The model under review builds one solid part; all positions refer to its coordinate system, in mm. A direction names the side the tool comes from. Give positions to 0.01 mm unless a question says otherwise; leave off trailing zeros. Write each loop counter-clockwise with the first axis right and the second up, starting at its lowest first coordinate (ties: lowest second). Pieces come first, ordered by that corner, then holes. Notation, with made-up numbers: (54, 39) - (65, 39) arc R24 cw to (65, 66) - close; hole circle Ø5 at (-40, 1.5). An arc over 180 degrees is marked (long way). Write item = value, one per line.
```python
from build123d import *

# Parameters (mm, degrees)
F0_W      = 124
F0_H      = 240
F1_DEPTH  = 18.5
F2_R      = 39
F2_R_2    = 17.85
F3_DEPTH  = 18.501
F5_DEPTH  = 13.5
F7_R      = 3.55
F8_DEPTH  = 2.6
F9_W      = 39.5
F9_H      = 42.75
F10_DEPTH = 6.5
F11_R     = 3


with BuildPart() as f1:
    # F0 (on Front) → F1 (new body)
    with BuildSketch(Plane.XZ):
        with Locations((62, -120)):
            Rectangle(F0_W, F0_H)
    extrude(amount=F1_DEPTH)

    # F2 (on face) → F3 (cut, through all)
    with BuildSketch(Plane(origin=(0, 0, 0), x_dir=(-1, 0, 0), z_dir=(0, 1, 0))):
        with Locations((-62, -62)):
            Circle(F2_R)
        with Locations((-62, -125.85)):
            Circle(F2_R_2)
    extrude(amount=-F3_DEPTH, mode=Mode.SUBTRACT)

    # F4 (on face) → F5 (cut)
    with BuildSketch(Plane(origin=(0, 0, 0), x_dir=(-1, 0, 0), z_dir=(0, 1, 0))):
        with BuildLine():
            ThreePointArc((-24.970595501, -99.029404499), (-17, -62), (-24.970595501, -24.970595501))
            ThreePointArc((-24.970595501, -24.970595501), (-62, -17), (-99.029404499, -24.970595501))
            ThreePointArc((-99.029404499, -24.970595501), (-107, -62), (-99.029404499, -99.029404499))
            ThreePointArc((-99.029404499, -99.029404499), (-62, -107), (-24.970595501, -99.029404499))
        make_face()
    extrude(amount=-F5_DEPTH, mode=Mode.SUBTRACT)

    # F7 (on offset) → F8 (cut)
    with BuildSketch(Plane.XZ.offset(13.5)):
        with Locations((29.1195346748, -29.1195346748)):
            Circle(F7_R)
        with Locations((29.1195346748, -94.8804653252)):
            Circle(F7_R)
        with Locations((94.8804653252, -94.8804653252)):
            Circle(F7_R)
        with Locations((94.8804653252, -29.1195346748)):
            Circle(F7_R)
    extrude(amount=F8_DEPTH, mode=Mode.SUBTRACT)

    # F9 (on face) → F10 (cut)
    with BuildSketch(Plane(origin=(0, 0, 0), x_dir=(-1, 0, 0), z_dir=(0, 1, 0))):
        with Locations((-62, -124.225)):
            Rectangle(F9_W, F9_H)
    extrude(amount=-F10_DEPTH, mode=Mode.SUBTRACT)

    # F11
    f11_edges = [f1.edges().sort_by_distance(p)[0] for p in [
        (81.75, -3.25, -145.6),
        (42.25, -3.25, -145.6),
        (99.029404, -6.75, -99.029404),
        (24.970596, -6.75, -99.029404),
        (24.970596, -6.75, -24.970596),
        (99.029404, -6.75, -24.970596),
    ]]
    fillet(f11_edges, radius=F11_R)


solid = f1.part
```
1. Take a section at C-C on x = 39.5. Give the boundary of the cut face in (y, z).
Findings below:
outline = (-18.5, -240) - (0, -240) - (0, -104.14) - (-13.5, -104.14) - (-13.5, -93.86) - (-18.5, -93.86) - close; (-18.5, -30.14) - (-13.5, -30.14) - (-13.5, -19.86) - (0, -19.86) - (0, 0) - (-18.5, 0) - close
2. For line 1 (Z direction, x = 62, y = -14.25); line 2 (Z direction, x = 78.5, y = -9.75); line 3 (Z direction, x = 93, y = -3), list the stretches that pass through material, from the lowest coordinate up. Write a range as from..to.
Findings below:
line_1 = -240..-143.7, -108..-101, -23..0
line_2 = -240..-132.66, -119.04..-105.47, -18.53..0
line_3 = -240..-101.49, -22.51..0
3. Take a section at A-A on z = -62. Give the boundary of the cut face in (x, y), and give its area (3 significant figures).
Findings below:
outline = (0, -18.5) - (23, -18.5) - (23, -13.5) - (17, -13.5) - (17, 0) - (0, 0) - close; (101, -18.5) - (124, -18.5) - (124, 0) - (107, 0) - (107, -13.5) - (101, -13.5) - close
area = 689 mm²
4. Take a section at B-B on x = 62. Give the boundary of the cut face in (y, z), and give its area (3 significant figures).
Findings below:
outline = (-18.5, -240) - (0, -240) - (0, -145.6) - (-6.5, -145.6) - (-6.5, -143.7) - (-18.5, -143.7) - close; (-18.5, -108) - (-6.5, -108) - (-6.5, -107) - (-13.5, -107) - (-13.5, -101) - (-18.5, -101) - close; (-18.5, -23) - (-13.5, -23) - (-13.5, -17) - (0, -17) - (0, 0) - (-18.5, 0) - close
area = 2,160 mm²
5. Draft analysis for pull direction X (two halves, no side actions). For faces 3 (the cylindrical face through (44.004, -15.965, -96.6)), 4 (the flat face through (34, 0, -145)), 5 (the flat face through (124, -9, -122)), state which applies: +X half, -X half, draft (parallel to the pull), parting line (faces both ways), or undercut.
Findings below:
face_3 = undercut
face_4 = draft
face_5 = +X half
6. Machinability: for faces 1 (the flat face through (61, -9, -240)), 2 (the cylindrical face through (62.5, -8.2, -107)), which of the approach directions +Z, -Z, +X, -X, +Y, -Y give a long, thin tool a straight path to every point of the face, cutting with its end or side? Answer none if there is none.
Findings below:
face_1 = -Z, +X, -X, +Y, -Y
face_2 = +Y
7. Insertion check: P1, Ø3.5, axis at x = 29.5, z = -93, coming from the +Y side; P2, Ø8, axis at x = 74.5, z = -110.5, coming from the +Y side; P3, Ø2, axis at x = 96.5, z = -29.5, coming from the +Y side. Each pin has a flat end and moves straight along its axis. Give the tip position at first contact, or say it passes through.
Findings below:
P1 = -13.5
P2 = -6.5
P3 = -16.1
